For this review, take the finished solid that the model builds, in its own axes (mm). Face numbers are marked on the shaded views. A direction names the side the tool comes from. Coordinates: 2 decimals unless noted, no trailing zeros. Order: outer loops, then holes, each group sorted by start corner. A loop starts at its lowest first (then second) coordinate and runs counter-clockwise, first axis right, second up. Notation, with made-up numbers: M -25,14.25 L 11,14.25 A21 ccw 11,46.25 Z; hole C 62.25,87 d3. An arc over 180 degrees is marked long. Use one line per item in the form item = value. Start each with the question number.
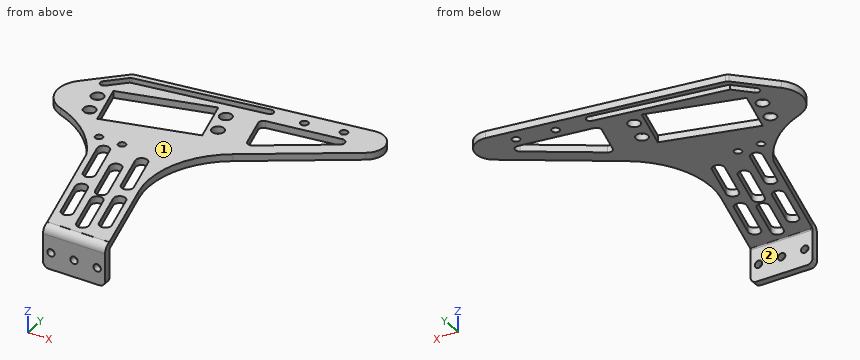
```python
from build123d import *

# Parameters (mm, degrees)
EXTRUDE_1_DEPTH              = 3
EXTRUDE_2_DEPTH              = 120
CUT_EXTRUDE_1_DEPTH          = 195.561044405
SKETCH_9_R                   = 0.555167329
CUT_EXTRUDE_3_DEPTH          = 10
HOLE_WIZARD_M5_1_D           = 4.2
HOLE_WIZARD_M5_1_DEPTH       = 12.4
HOLE_WIZARD_M5_1_CSINK_D     = 5.05
HOLE_WIZARD_M5_1_CSINK_ANGLE = 90
HOLE_WIZARD_M5_1_TIP         = 1.2618073
SKETCH_12_R                  = 0.419228838
SKETCH_12_R_2                = 0.457437139
CUT_EXTRUDE_4_DEPTH          = 10
HOLE_WIZARD_M3_1_D           = 2.5
HOLE_WIZARD_M3_1_DEPTH       = 7.5
HOLE_WIZARD_M3_1_CSINK_D     = 3.05
HOLE_WIZARD_M3_1_CSINK_ANGLE = 90
HOLE_WIZARD_M3_1_TIP         = 0.751075774
SKETCH_31_W                  = 27
SKETCH_31_H                  = 3
CUT_EXTRUDE_7_DEPTH          = 18
SKETCH_42_R                  = 1.6
SKETCH_42_R_2                = 2.6
CUT_EXTRUDE_9_DEPTH          = 18
SKETCH_43_R                  = 1.65
CUT_EXTRUDE_10_DEPTH         = 18
SM_BASE_FLANGE_2_DEPTH       = 27
CUT_EXTRUDE_11_DEPTH         = 10
SKETCH_54_R                  = 1.6
CUT_EXTRUDE_12_DEPTH         = 10
CUT_EXTRUDE_13_DEPTH         = 153.01995181
CUT_EXTRUDE_14_DEPTH         = 153.01995181


# Sheet-metal steps are written as plain solids
with BuildPart() as part:
    # 草图2 → 凸台-拉伸1 (new body)
    with BuildSketch(Plane(origin=(0, 0, 0), x_dir=(1, 0, 0), z_dir=(0, 1, 0))):
        with BuildLine():
            Line((0, 0), (27, 0))
            Line((27, 0), (27, -16))
            ThreePointArc((27, -16), (26.414213562, -17.414213562), (25, -18))
            Line((25, -18), (2, -18))
            ThreePointArc((2, -18), (0.585786438, -17.414213562), (0, -16))
            Line((0, -16), (0, 0))
        make_face()
    extrude(amount=EXTRUDE_1_DEPTH)

    # Sketch 3 → 凸台-拉伸2 (add)
    with BuildSketch(Plane(origin=(0, 3, 0), x_dir=(1, 0, 0), z_dir=(0, 1, 0))):
        Polygon((0, 0), (150, 0), (150, -3), (-100, -3), (-100, 0), align=None)
    extrude(amount=EXTRUDE_2_DEPTH)

    # Sketch 4 → 切除-拉伸1 (cut, through all)
    with BuildSketch(Plane.XY.offset(3)):
        with BuildLine():
            Line((-27.465625599, 108.090395999), (81.955038276, 122.874558425))
            ThreePointArc((81.955038276, 122.874558425), (87.311898998, 119.659835192), (85.350748847, 113.728200311))
            Line((85.350748847, 113.728200311), (33.001315422, 79.678206183))
            ThreePointArc((33.001315422, 79.678206183), (18.570908538, 61.838352676), (17.374177378, 38.924059091))
            Line((17.374177378, 38.924059091), (27, 3))
            Line((27, 3), (150, 3))
            Line((150, 3), (150, 123))
            Line((150, 123), (-100, 123))
            Line((-100, 123), (-100, 3))
            Line((-100, 3), (0, 3))
            Line((0, 3), (-12.940952255, 51.296291314))
            ThreePointArc((-12.940952255, 51.296291314), (-23.474992402, 64.922058411), (-38.267104772, 73.743676313))
            ThreePointArc((-38.267104772, 73.743676313), (-45.866257029, 82.424841396), (-42.634405947, 93.500259258))
            Line((-42.634405947, 93.500259258), (-28.612046307, 107.522618899))
            ThreePointArc((-28.612046307, 107.522618899), (-28.085458288, 107.900644409), (-27.465625599, 108.090395999))
        make_face()
    extrude(amount=-CUT_EXTRUDE_1_DEPTH, mode=Mode.SUBTRACT)

    # 草图9 → 切除-拉伸3 (cut)
    with BuildSketch(Plane.XY.offset(3)):
        with Locations((-28.427787155, 78.364928444)):
            Circle(SKETCH_9_R)
        with Locations((-31.021767983, 88.02263332)):
            Circle(SKETCH_9_R)
        with Locations((19.37785198, 91.205133539)):
            Circle(SKETCH_9_R)
        with Locations((16.783871152, 100.862838415)):
            Circle(SKETCH_9_R)
        Polygon((-22.719980027, 74.461924756), (-28.037640723, 94.260219752), (11.076064024, 104.765842103), (16.39372472, 84.967547107), align=None)
    extrude(amount=-CUT_EXTRUDE_3_DEPTH, mode=Mode.SUBTRACT)

    # M5 螺纹孔1
    with Locations(Plane.XY.offset(3)):
        with Locations((-31.021767983, 88.02263332), (-28.427787155, 78.364928444), (16.783871152, 100.862838415), (19.37785198, 91.205133539)):
            CounterSinkHole(HOLE_WIZARD_M5_1_D / 2, HOLE_WIZARD_M5_1_CSINK_D / 2, depth=HOLE_WIZARD_M5_1_DEPTH, counter_sink_angle=HOLE_WIZARD_M5_1_CSINK_ANGLE)
            with Locations((0, 0, -(HOLE_WIZARD_M5_1_DEPTH + HOLE_WIZARD_M5_1_TIP / 2))):  # 118° drill point
                Cone(0, HOLE_WIZARD_M5_1_D / 2, HOLE_WIZARD_M5_1_TIP, mode=Mode.SUBTRACT)

    # 草图12 → 切除-拉伸4 (cut)
    with BuildSketch(Plane.XY.offset(3)):
        with Locations((-5.383085829, 63.900528175)):
            Circle(SKETCH_12_R)
        with Locations((-15.383085829, 63.900528175)):
            Circle(SKETCH_12_R_2)
        Polygon((-27.731348581, 94.083626651), (10.899470923, 104.45954996), (16.087432577, 85.144140208), (-22.543386926, 74.768216899), align=None)
    extrude(amount=-CUT_EXTRUDE_4_DEPTH, mode=Mode.SUBTRACT)

    # M3 螺纹孔1
    with Locations(Plane.XY.offset(3)):
        with Locations((-15.383085829, 63.900528175), (-5.383085829, 63.900528175)):
            CounterSinkHole(HOLE_WIZARD_M3_1_D / 2, HOLE_WIZARD_M3_1_CSINK_D / 2, depth=HOLE_WIZARD_M3_1_DEPTH, counter_sink_angle=HOLE_WIZARD_M3_1_CSINK_ANGLE)
            with Locations((0, 0, -(HOLE_WIZARD_M3_1_DEPTH + HOLE_WIZARD_M3_1_TIP / 2))):  # 118° drill point
                Cone(0, HOLE_WIZARD_M3_1_D / 2, HOLE_WIZARD_M3_1_TIP, mode=Mode.SUBTRACT)

    # 草图31 → 切除-拉伸7 (cut)
    with BuildSketch(Plane(origin=(0, 0, 0), x_dir=(-1, 0, 0), z_dir=(0, 0, -1))):
        with Locations((-13.5, 1.5)):
            Rectangle(SKETCH_31_W, SKETCH_31_H)
    extrude(amount=-CUT_EXTRUDE_7_DEPTH, mode=Mode.SUBTRACT)

    # 草图42 → 切除-拉伸9 (cut)
    with BuildSketch(Plane.XY.offset(3)):
        with Locations((-15.383085829, 63.900528175)):
            Circle(SKETCH_42_R)
        with Locations((-5.383085829, 63.900528175)):
            Circle(SKETCH_42_R)
        with Locations((-28.427787155, 78.364928444)):
            Circle(SKETCH_42_R_2)
        with Locations((-31.021767983, 88.02263332)):
            Circle(SKETCH_42_R_2)
        with Locations((16.783871152, 100.862838415)):
            Circle(SKETCH_42_R_2)
        with Locations((19.37785198, 91.205133539)):
            Circle(SKETCH_42_R_2)
        with BuildLine():
            Line((11.987750487, 29.73961726), (16.646493299, 12.352952387))
            ThreePointArc((16.646493299, 12.352952387), (19.708355477, 10.585185434), (21.47612243, 13.647047613))
            Line((21.47612243, 13.647047613), (16.817379618, 31.033712486))
            ThreePointArc((16.817379618, 31.033712486), (13.75551744, 32.801479439), (11.987750487, 29.73961726))
        make_face()
        with BuildLine():
            Line((-11.823601663, 56.785540397), (-7.164858851, 39.398875523))
            ThreePointArc((-7.164858851, 39.398875523), (-4.102996672, 37.63110857), (-2.335229719, 40.692970749))
            Line((-2.335229719, 40.692970749), (-6.993972531, 58.079635622))
            ThreePointArc((-6.993972531, 58.079635622), (-10.05583471, 59.847402575), (-11.823601663, 56.785540397))
        make_face()
        with BuildLine():
            Line((-4.5766684, 29.73961726), (0.082074412, 12.352952387))
            ThreePointArc((0.082074412, 12.352952387), (3.14393659, 10.585185434), (4.911703543, 13.647047613))
            Line((4.911703543, 13.647047613), (0.252960732, 31.033712486))
            ThreePointArc((0.252960732, 31.033712486), (-2.808901447, 32.801479439), (-4.5766684, 29.73961726))
        make_face()
        with BuildLine():
            Line((-1.301722379, 48.426978761), (3.358398139, 31.035172218))
            ThreePointArc((3.358398139, 31.035172218), (6.420260317, 29.267405265), (8.18802727, 32.329267444))
            Line((8.18802727, 32.329267444), (3.527906752, 49.721073986))
            ThreePointArc((3.527906752, 49.721073986), (0.466044574, 51.488840939), (-1.301722379, 48.426978761))
        make_face()
        with BuildLine():
            Line((4.740817224, 56.785540397), (9.399560036, 39.398875523))
            ThreePointArc((9.399560036, 39.398875523), (12.461422214, 37.63110857), (14.229189167, 40.692970749))
            Line((14.229189167, 40.692970749), (9.570446355, 58.079635622))
            ThreePointArc((9.570446355, 58.079635622), (6.508584177, 59.847402575), (4.740817224, 56.785540397))
        make_face()
        with BuildLine():
            Line((4.911312409, 25.23961726), (9.570055221, 7.852952387))
            ThreePointArc((9.570055221, 7.852952387), (12.6319174, 6.085185434), (14.399684353, 9.147047613))
            Line((14.399684353, 9.147047613), (9.740941541, 26.533712486))
            ThreePointArc((9.740941541, 26.533712486), (6.679079362, 28.301479439), (4.911312409, 25.23961726))
        make_face()
    extrude(amount=-CUT_EXTRUDE_9_DEPTH, mode=Mode.SUBTRACT)

    # 草图43 → 切除-拉伸10 (cut)
    with BuildSketch(Plane.XY.offset(3)):
        with Locations((43.853289388, 112.252662001)):
            Circle(SKETCH_43_R)
        with Locations((59.70921469, 114.395004835)):
            Circle(SKETCH_43_R)
        with BuildLine():
            Line((-34.854948443, 98.060205677), (-27.783880632, 105.131273489))
            ThreePointArc((-27.783880632, 105.131273489), (-27.372130398, 105.428939436), (-26.887815625, 105.582505293))
            Line((-26.887815625, 105.582505293), (28.617983545, 113.835264655))
            ThreePointArc((28.617983545, 113.835264655), (30.435892042, 112.487967844), (29.088595231, 110.670059347))
            Line((29.088595231, 110.670059347), (-25.894680467, 102.494990254))
            Line((-25.894680467, 102.494990254), (-32.592206744, 95.797463977))
            ThreePointArc((-32.592206744, 95.797463977), (-34.854948443, 95.797463977), (-34.854948443, 98.060205677))
        make_face()
    extrude(amount=-CUT_EXTRUDE_10_DEPTH, mode=Mode.SUBTRACT)

    # 草图55 → 切除-拉伸13 (cut, through all)
    with BuildSketch(Plane.XY.offset(3)):
        with BuildLine():
            Line((61.704894996, 110.047634391), (30.943691051, 105.891393518))
            ThreePointArc((30.943691051, 105.891393518), (29.546325951, 105.017215559), (29.27994293, 103.39060669))
            Line((29.27994293, 103.39060669), (32.904446455, 89.896140965))
            ThreePointArc((32.904446455, 89.896140965), (34.120486844, 88.547302554), (35.926478804, 88.738384548))
            Line((35.926478804, 88.738384548), (63.063179225, 106.389091146))
            ThreePointArc((63.063179225, 106.389091146), (63.847639285, 108.761745098), (61.704894996, 110.047634391))
        make_face()
    extrude(amount=-CUT_EXTRUDE_13_DEPTH, mode=Mode.SUBTRACT)

    # 草图56 → 切除-拉伸14 (cut, through all)
    with BuildSketch(Plane.XY.offset(3)):
        with BuildLine():
            Line((85.350748847, 113.728200311), (74.167295897, 106.45407178))
            ThreePointArc((74.167295897, 106.45407178), (77.30513614, 115.944687589), (68.734158983, 121.088244762))
            Line((68.734158983, 121.088244762), (81.955038276, 122.874558425))
            ThreePointArc((81.955038276, 122.874558425), (87.311898998, 119.659835192), (85.350748847, 113.728200311))
        make_face()
    extrude(amount=-CUT_EXTRUDE_14_DEPTH, mode=Mode.SUBTRACT)


with BuildPart() as body_2:
    # 草图44 → 基体-法兰2 (new body)
    with BuildSketch(Plane(origin=(0, 0, 0), x_dir=(0, 0, -1), z_dir=(1, 0, 0))):
        with BuildLine():
            Line((-3, 6), (-3, 3.5))
            ThreePointArc((-3, 3.5), (-1.974873734, 1.025126266), (0.5, 0))
            Line((0.5, 0), (14.96623469, 0))
            Line((14.96623469, 0), (14.96623469, 3))
            Line((14.96623469, 3), (0.5, 3))
            ThreePointArc((0.5, 3), (0.146446609, 3.146446609), (0, 3.5))
            Line((0, 3.5), (0, 6))
            Line((0, 6), (-3, 6))
        make_face()
    extrude(amount=SM_BASE_FLANGE_2_DEPTH)

    # 草图53 → 切除-拉伸11 (cut)
    with BuildSketch(Plane.XY.offset(3)):
        Polygon((27, 3), (26.196152423, 6), (27, 6), align=None)
    extrude(amount=-CUT_EXTRUDE_11_DEPTH, mode=Mode.SUBTRACT)

    # 草图54 → 切除-拉伸12 (cut)
    with BuildSketch(Plane(origin=(0, 3, 0), x_dir=(1, 0, 0), z_dir=(0, 1, 0))):
        with Locations(Location((3.45, 7.733117345, 0), (0, 0, 270))):
            Circle(SKETCH_54_R)
        with Locations(Location((23.55, 7.733117345, 0), (0, 0, 270))):
            Circle(SKETCH_54_R)
        with Locations(Location((13.5, 7.733117345, 0), (0, 0, 270))):
            Circle(SKETCH_54_R)
        with BuildLine():
            Line((24.5, 14.96623469), (27, 14.96623469))
            Line((27, 14.96623469), (27, 12.46623469))
            ThreePointArc((27, 12.46623469), (26.267766953, 14.234001643), (24.5, 14.96623469))
        make_face()
        with BuildLine():
            Line((0, 14.96623469), (2.5, 14.96623469))
            ThreePointArc((2.5, 14.96623469), (0.732233047, 14.234001643), (0, 12.46623469))
            Line((0, 12.46623469), (0, 14.96623469))
        make_face()
    extrude(amount=-CUT_EXTRUDE_12_DEPTH, mode=Mode.SUBTRACT)


with BuildPart() as part_1:
    add(part.part)

    # Combine 1: union body 2
    add(body_2.part)


solid = part_1.part
```
1. For pin 1 Ø5 at (x, z) = (22, -6.5) entering from +Y; pin 2 Ø4 at (y, z) = (1.5, -6) entering from -X; pin 3 Ø5 at (x, z) = (12.5, -0.5) entering from +Y, all flat-tipped, find the tip position at first contact; note any pin that passes through.
2. To check wall thickness, follow line 1 (Y direction, x = 15.5, z = -13.5); line 2 (X direction, y = 28.5, z = 1.75); line 3 (X direction, y = 31.5, z = 1.5). State the ranges of each line that lie inside material, in increasing order.
3. Consider section C-C, the plane z = -2.5. Write out the cut boundary in (x, y), plus the area to 3 significant figures.
4. Consider section A-A, the plane y = 18.5. Write out the cut boundary in (x, z), plus the area to 3 significant figures.
5. Consider section B-B, the plane x = 53.5. Write out the cut boundary in (y, z), plus the area to 3 significant figures.
6. Tool access review of the marked faces 1 and 2: name each direction out of +Z, -Z, +X, -X, +Y, -Y from which nothing blocks a thin tool from reaching the whole face with its end or side.
Answers follow:
q1.pin_1 = 3
q1.pin_2 = 0
q1.pin_3 = 113.82
q2.line_1 = 0 to 3
q2.line_2 = -6.83 to -4.24, 0.93 to 12.32, 17.5 to 20.17
q2.line_3 = -7.64 to -4.4, 0.08 to 3.23, 8.27 to 12.16, 16.64 to 19.36
q3.outline = M 0,0 L 27,0 L 27,3 L 0,3 Z
q3.area = 81.0 mm²
q4.outline = M -4.15,0 L -1.57,0 L -1.57,3 L -4.15,3 Z; M 3.61,0 L 6.72,0 L 6.72,3 L 3.61,3 Z; M 11.89,0 L 15,0 L 15,3 L 11.89,3 Z; M 20.18,0 L 22.85,0 L 22.85,3 L 20.18,3 Z
q4.area = 34.4 mm²
q5.outline = M 93.01,0 L 100.17,0 L 100.17,3 L 93.01,3 Z; M 108.94,0 L 119.03,0 L 119.03,3 L 108.94,3 Z
q5.area = 51.7 mm²
q6.face_1 = +Z, +X, -X, +Y, -Y
q6.face_2 = -Z, +X, -X, +Y
